For this review, take the finished solid that the model builds, in its own axes (mm). A direction names the side the tool comes from. Round coordinates to 2 decimals unless told otherwise and drop trailing zeros. Loops run counter-clockwise (first coordinate to the right, second up) from the corner with the lowest first, then second, coordinate; pieces in that order, holes last.
```python
from build123d import *

# Parameters (mm, degrees)
BOSS_EXTRUDE1_DEPTH     = 6.35
SKETCH1_3_R             = 10
SKETCH1_3_R_2           = 4
BOSS_EXTRUDE2_DEPTH     = 18.7
CUT_EXTRUDE1_DEPTH      = 55.130565784
CUT_EXTRUDE1_DEPTH_BACK = 55.130565784
SKETCH3_R               = 12.5
CUT_EXTRUDE3_DEPTH      = 55.130565784
CUT_EXTRUDE3_DEPTH_BACK = 55.130565784
SKETCH4_R               = 12.5
BOSS_EXTRUDE3_START     = -5
BOSS_EXTRUDE3_DEPTH     = 5


with BuildPart() as part:
    # Sketch1 → Boss-Extrude1 (new body)
    with BuildSketch(Plane(origin=(0, 0, 0), x_dir=(1, 0, 0), z_dir=(0, 1, 0))):
        with BuildLine():
            Line((30.820134884, -20.651845529), (30.820134884, 40.348154471))
            Line((30.820134884, 40.348154471), (1.797901548, 40.348154471))
            ThreePointArc((1.797901548, 40.348154471), (8.347755505, 37.163141176), (11.000000332, 30.380037615))
            ThreePointArc((11.000000332, 30.380037615), (7.256441333, 22.578951408), (-1.171388868, 20.618630496))
            Line((-1.171388868, 20.618630496), (-13.427648664, -20.651845529))
            Line((-13.427648664, -20.651845529), (30.820134884, -20.651845529))
        make_face()
    extrude(amount=BOSS_EXTRUDE1_DEPTH)

    # Sketch1_3 → Boss-Extrude2 (add)
    with BuildSketch(Plane(origin=(0, 0, 0), x_dir=(1, 0, 0), z_dir=(0, 1, 0))):
        with Locations(Location((1.000000332, 30.380037615, 0), (0, 0, 85.423497978))):
            Circle(SKETCH1_3_R)
        with Locations(Location((1.000000332, 30.380037615, 0), (0, 0, 270))):
            Circle(SKETCH1_3_R_2, mode=Mode.SUBTRACT)
    extrude(amount=BOSS_EXTRUDE2_DEPTH)

    # Sketch3 → Cut-Extrude1 (cut, two sides: drawn at the far end of the back side and taken through both)
    with BuildSketch(Plane.XY.offset(-CUT_EXTRUDE1_DEPTH_BACK)):
        with Locations((42.910187614, 3.175)):
            Circle(SKETCH3_R)
    extrude(amount=CUT_EXTRUDE1_DEPTH + CUT_EXTRUDE1_DEPTH_BACK, mode=Mode.SUBTRACT)

    # Sketch4 → Cut-Extrude3 (cut, two sides: drawn at the far end of the back side and taken through both)
    with BuildSketch(Plane(origin=(0, 0, 0), x_dir=(0, 0, -1), z_dir=(1, 0, 0)).offset(-CUT_EXTRUDE3_DEPTH_BACK)):
        with Locations((-32.741898259, 3.175)):
            Circle(SKETCH4_R)
    extrude(amount=CUT_EXTRUDE3_DEPTH + CUT_EXTRUDE3_DEPTH_BACK, mode=Mode.SUBTRACT)

    # Sketch5 → Boss-Extrude3 (add)
    with BuildSketch(Plane(origin=(0, 18.7, 0), x_dir=(1, 0, 0), z_dir=(0, 1, 0)).offset(BOSS_EXTRUDE3_START)):
        with BuildLine():
            ThreePointArc((9.716620703, 25.478963312), (-1.533159384, 20.706201672), (-8.999999668, 30.380037615))
            Line((-8.999999668, 30.380037615), (-8.999999668, -41.582926526))
            Line((-8.999999668, -41.582926526), (28.938924754, -41.582926526))
            ThreePointArc((28.938924754, -41.582926526), (32.982787431, -17.815786501), (44.256083353, 3.494834546))
            Line((44.256083353, 3.494834546), (44.256083353, 19.094758402))
            Line((44.256083353, 19.094758402), (9.716620703, 25.478963312))
        make_face()
        Polygon((17.594978634, -31.436293162), (0, -31.436293162), (0, 0), (6.242345966, 0), align=None, mode=Mode.SUBTRACT)
        Polygon((28.816009284, -1.183711765), (11.455147871, 8.481691767), (15.20184924, 18.147095298), (36.949007186, 13.314393532), align=None, mode=Mode.SUBTRACT)
    extrude(amount=BOSS_EXTRUDE3_DEPTH)


solid = part.part
```
(1) The part is to be moulded in two halves that separate along X. For faces 1 (the cylindrical face through (30.41, 3.22, -10.28)), 2 (the flat face through (20.26, 16.16, -3.58)), 3 (the flat face through (-7.214, 3.131, -0.272)), 4 (the flat face through (9, 16, 31.436)), say which applies: pulls with the +X half, pulls with the -X half, needs draft (parallel to the pull), parting line crosses it, or undercut.
(2) Add section C-C (y = 8.25). Give the boundary of the cut face in (x, z).
(3) Insertion check: pin 1 Ø4 at (y, z) = (17, 16.5) entering from -X; pin 2 Ø10 at (y, z) = (7.5, 22.5) entering from +X; pin 3 Ø10 at (x, y) = (29, 9.5) entering from +Z; pin 4 Ø4 at (x, y) = (13.5, 9.5) entering from -Z. Each pin has a flat end and moves straight along its axis. Give the tip position at first contact, or say it passes through.
(4) Add section D-D (y = 4.25). Give the boundary of the cut face in (x, z).
(5) For faces 5 (the cylindrical face through (-6.976, 9.219, -36.412)), 6 (the flat face through (0, 16, 16)), 7 (the flat face through (10, 18.7, 2)), list the 3-axis set-ups (+Z, -Z, +X, -X, +Y, -Y) from which the entire face can be reached by the end or side of a thin tool; tool diameter is ignored.
(6) Add section A-A (z = 23). Give the boundary of the cut face in (x, y).
(7) For L1, parallel to Y at x = 10.5, z = 5; L2, parallel to Z at x = 12, y = 3.5; L3, parallel to Y at x = 23.5, z = -25, list the stretches that pass through material, from the lowest coordinate up.
(8) Add section B-B (y = 15.25). Give the boundary of the cut face in (x, z).
Outcome:
1. face 1: pulls with the +X half
1. face 2: undercut
1. face 3: pulls with the -X half
1. face 4: undercut
2. outline: circle Ø20 at (1, -30.38); hole circle Ø8 at (1, -30.38)
3. pin 1: stops at x = -9
3. pin 2: stops at x = 30.82
3. pin 3: stops at z = 41.58
3. pin 4: passes through
4. outline: (-13.32, 20.29) - (-1.17, -20.62) arc R10 ccw to (1.8, -40.35) - (30.46, -40.35) - (30.46, 20.29) - close; hole circle Ø8 at (1, -30.38)
5. face 5: none
5. face 6: +Y
5. face 7: +Z, -Z, +X, -X, +Y
6. outline: (-9, 13.7) - (0, 13.7) - (0, 18.7) - (-9, 18.7) - close; (14.55, 13.7) - (31.42, 13.7) - (31.42, 18.7) - (14.55, 18.7) - close
7. L1: y = 0 to 6.35, 13.7 to 18.7
7. L2: z = -40.35 to 20.25
7. L3: y = 0 to 6.35
8. outline: (-9, -30.38) arc R10 ccw (long way) to (9.72, -25.48) - (44.26, -19.09) - (44.26, -3.49) arc R76.12 cw to (28.94, 41.58) - (-9, 41.58) - close; hole circle Ø8 at (1, -30.38); hole (0, 0) - (6.24, 0) - (17.59, 31.44) - (0, 31.44) - close; hole (11.46, -8.48) - (15.2, -18.15) - (36.95, -13.31) - (28.82, 1.18) - close
